Read the model definition and answer for the solid it produces. Units are mm, in the model's axes. Face numbers are marked on the shaded views. A direction names the side the tool comes from. Give positions to 0.01 mm unless a question says otherwise; leave off trailing zeros. Write each loop counter-clockwise with the first axis right and the second up, starting at its lowest first coordinate (ties: lowest second). Pieces come first, ordered by that corner, then holes. Notation, with made-up numbers: M 28.5,80.25 L 79.5,80.25 A23 cw 79.5,88.25 Z; hole C 16.5,6 d3. An arc over 180 degrees is marked long. Put each result on its own line as item: value.
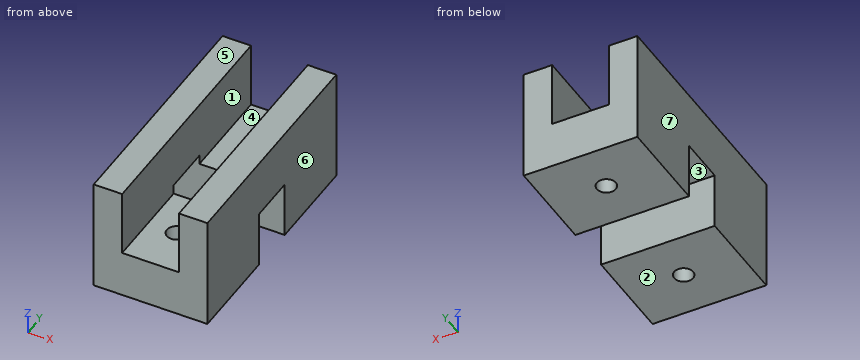
from build123d import *

# Parameters (mm, degrees)
BOSS_EXTRUDE1_DEPTH = 30
SKETCH2_W           = 30
SKETCH2_H           = 35
CUT_EXTRUDE1_DEPTH  = 133.003787824
SKETCH3_R           = 5
CUT_EXTRUDE2_DEPTH  = 78.661122835


with BuildPart() as part:
    # Sketch1 → Boss-Extrude1 (new, symmetric)
    with BuildSketch(Plane.YZ):
        Polygon((-62.5, 30), (-62.5, -30), (-12.5, -30), (-12.5, 0), (12.5, 0), (12.5, -30), (62.5, -30), (62.5, 30), align=None)
    extrude(amount=BOSS_EXTRUDE1_DEPTH, both=True)

    # Sketch2 → Cut-Extrude1 (cut, through all)
    with BuildSketch(Plane(origin=(0, 62.5, 0), x_dir=(-1, 0, 0), z_dir=(0, 1, 0))):
        with Locations((0, 12.5)):
            Rectangle(SKETCH2_W, SKETCH2_H)
    extrude(amount=-CUT_EXTRUDE1_DEPTH, mode=Mode.SUBTRACT)

    # Sketch3 → Cut-Extrude2 (cut, through all)
    with BuildSketch(Plane.XY.offset(-5)):
        with Locations((0, -37.5)):
            Circle(SKETCH3_R)
        with Locations((0, 37.5)):
            Circle(SKETCH3_R)
    extrude(amount=-CUT_EXTRUDE2_DEPTH, mode=Mode.SUBTRACT)


solid = part.part
(1) For a pull along X with two mould halves and no side action, classify the marked faces 4, 5, 6 and 7 as +X half, -X half, draft (parallel to the pull), parting line (faces both ways), or undercut.
Result:
face 4: undercut
face 5: draft
face 6: +X half
face 7: -X half
(2) Section C-C on x = 6.5 is taken. Determine the outline of the cut face in (y, z), and give its area (3 significant figures).
Result:
outline: M -62.5,-30 L -12.5,-30 L -12.5,-5 L -62.5,-5 Z; M 12.5,-30 L 62.5,-30 L 62.5,-5 L 12.5,-5 Z
area: 2,500 mm²
(3) Section D-D on z = 18.5 is taken. Determine the outline of the cut face in (x, y).
Result:
outline: M -30,-62.5 L -15,-62.5 L -15,62.5 L -30,62.5 Z; M 15,-62.5 L 30,-62.5 L 30,62.5 L 15,62.5 Z
(4) Straight lines are drawn through the part: line 1 along Y through (x, z) = (0, -18); line 2 along X through (y, z) = (-37, -13); line 3 along X through (y, z) = (10, 13). For each, find the intervals that lie inside material, in ascending order. Write a range as from..to.
Result:
line 1: y = -62.5..-42.5, -32.5..-12.5, 12.5..32.5, 42.5..62.5
line 2: x = -30..-4.97, 4.97..30
line 3: x = -30..-15, 15..30
(5) Given pin 1 Ø1.5 at (x, y) = (-19, 10.5) entering from -Z; pin 2 Ø8 at (x, y) = (0, -37.5) entering from -Z; pin 3 Ø11.5 at (x, y) = (0, 37.5) entering from +Z, each flat-ended and moving along its own axis, determine where each tip first touches the part or whether it passes through.
Result:
pin 1: stops at z = 0
pin 2: passes through
pin 3: stops at z = -5
(6) Section B-B on y = 37.5 is taken. Determine the outline of the cut face in (x, z), and give its area (3 significant figures).
Result:
outline: M -30,-30 L -5,-30 L -5,-5 L -15,-5 L -15,30 L -30,30 Z; M 5,-30 L 30,-30 L 30,30 L 15,30 L 15,-5 L 5,-5 Z
area: 2,300 mm²
(7) Section A-A on z = -14 is taken. Determine the outline of the cut face in (x, y).
Result:
outline: M -30,-62.5 L 30,-62.5 L 30,-12.5 L -30,-12.5 Z; M -30,12.5 L 30,12.5 L 30,62.5 L -30,62.5 Z; hole C 0,-37.5 d10; hole C 0,37.5 d10
(8) Which of the six approach directions +Z, -Z, +X, -X, +Y, -Y give full straight-line access (tool end or side, diameter ignored) to the marked faces 1, 2 and 3?
Result:
face 1: +Z, +Y, -Y
face 2: -Z, +X, -X, +Y, -Y
face 3: -Z, +X, -X
